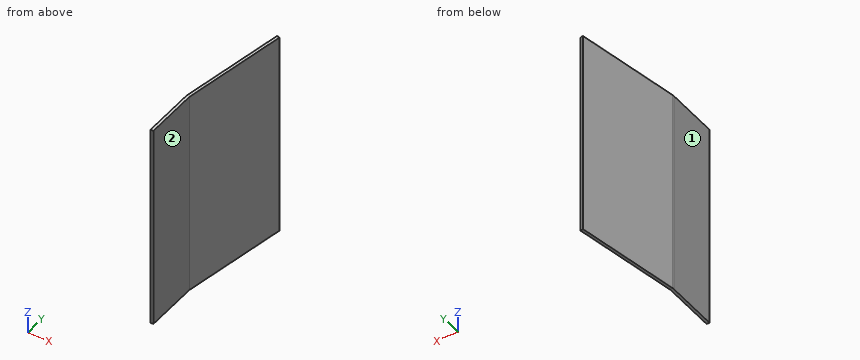
Autodesk Inventor part; units mm, degrees
ref_plane "YZ Plane" through (0, 0, 0) normal (1, 0, 0) x (0, 1, 0)
ref_plane "XZ Plane" through (0, 0, 0) normal (0, 1, 0) x (-1, 0, 0)
ref_plane "XY Plane" through (0, 0, 0) normal (0, 0, 1) x (1, 0, 0)
sketch "Sketch1" plane through (0, 0, 0) normal (0, 0, 1) x (1, 0, 0)
  line L0 (0, 0) -> (0, 118.2502)
  line L1 (0.3038, 121.7232) -> (41.6756, 356.3539)
  arc A0 (0.3038, 121.7232) -> (0, 118.2502) centre (20, 118.2502) ccw
  line L2 (47.9291, 355.2512) -> (6.35, 119.4444)
  line L3 (6.35, 119.4444) -> (6.35, 0)
  line L4 (41.6756, 356.3539) -> (47.9291, 355.2512)
  line L5 (0, 0) -> (6.35, 0)
  point P0 (0, 120)
  dimension "d0" = 170
  dimension "d1" = 120
  dimension "d2" = 240
  dimension "d3" = 20
  dimension "d4" = 6.35
extrude "Extrusion1" add sketch "Sketch1" along normal blind 450
properties part number "SteelBack"
For this review, take the finished solid that the model builds, in its own axes (mm). Face numbers are marked on the shaded views. A direction names the side the tool comes from. Round coordinates to 2 decimals unless told otherwise and drop trailing zeros. Loops run counter-clockwise (first coordinate to the right, second up) from the corner with the lowest first, then second, coordinate; pieces in that order, holes last.
Q1. Machinability: for the marked faces 1 and 2, which of the approach directions +Z, -Z, +X, -X, +Y, -Y give a long, thin tool a straight path to every point of the face, cutting with its end or side? Answer none if there is none.
Result sheet:
face 1: +Z, -Z, -X, +Y, -Y
face 2: +Z, -Z, +X, -Y
Q2. Add section C-C on x = 14.5. Write out the cut boundary in (y, z).
Result sheet:
outline: (165.67, 0) - (202.23, 0) - (202.23, 450) - (165.67, 450) - close
Q3. Add section A-A on z = 265. Write out the cut boundary in (x, y), plus the area to 3 significant figures.
Result sheet:
outline: (0, 0) - (6.35, 0) - (6.35, 119.44) - (47.93, 355.25) - (41.68, 356.35) - (0.3, 121.72) arc R19.99 ccw to (0, 118.25) - close
area: 2,280 mm2
Q4. To check wall thickness, follow line 1 along X through (y, z) = (35.5, 176.5); line 2 along X through (y, z) = (197, 108.5). State the ranges of each line that lie inside material, in increasing order.
Result sheet:
line 1: x = 0 to 6.35
line 2: x = 13.58 to 20.03
Q5. Insertion check: pin 1 Ø8 at (y, z) = (237, 251.5) entering from +X; pin 2 Ø2 at (y, z) = (83, 206) entering from +X; pin 3 Ø12 at (x, y) = (12.5, 103.5) entering from +Z; pin 4 Ø6 at (y, z) = (181, 93.5) entering from +X. Each pin has a flat end and moves straight along its axis. Give the tip position at first contact, or say it passes through.
Result sheet:
pin 1: stops at x = 27.78
pin 2: stops at x = 6.35
pin 3: passes through
pin 4: stops at x = 17.73
Q6. Add section B-B on y = 31.5. Write out the cut boundary in (x, z), plus the area to 3 significant figures.
Result sheet:
outline: (0, 0) - (6.35, 0) - (6.35, 450) - (0, 450) - close
area: 2,860 mm2
